Geometry: final body of the model. Coordinates: model frame, mm. Face numbers are marked on the shaded views. A direction names the side the tool comes from. Give positions to 0.01 mm unless a question says otherwise; leave off trailing zeros. Order: outer loops, then holes, each group sorted by start corner. A loop starts at its lowest first (then second) coordinate and runs counter-clockwise, first axis right, second up. Notation, with made-up numbers: (30, -13) -> (48, -13) arc R10 cw to (48, -7) -> close; hole circle Ø8 at (79, -24.75). An arc over 180 degrees is marked (long way). One line per item, written item: value. Start each with the question number.
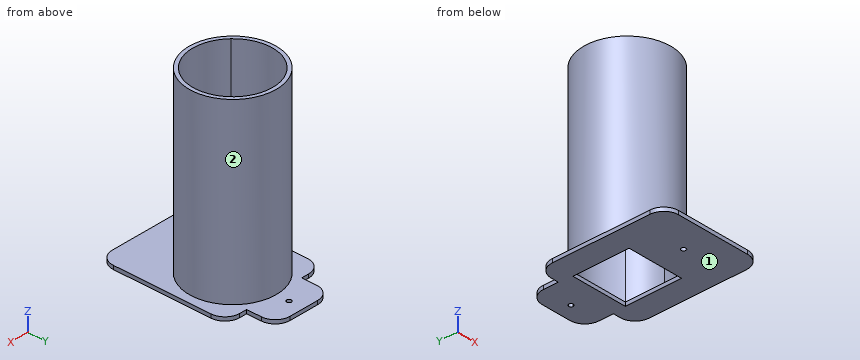
```python
from build123d import *

# Parameters (mm, degrees)
F0_W     = 24.13
F0_H     = 24.13
F0_W_2   = 44.45
F0_H_2   = 19.05
F0_R     = 1.016
F1_DEPTH = 1.5875
F2_R     = 6.35
F3_R     = 18.649987
F4_DEPTH = 76.2


with BuildPart() as f1:
    # F0 (on Top) → F1 (new body)
    with BuildSketch(Plane.XY):
        with BuildLine():
            Line((0, 17.78), (12.7, 17.78))
            Line((12.7, 17.78), (12.7, 30.48))
            Line((12.7, 30.48), (0, 30.48))
            Line((0, 30.48), (0, 25.146))
            ThreePointArc((0, 25.146), (0.71842, 24.84842), (1.016, 24.13))
            ThreePointArc((1.016, 24.13), (0.71842, 23.41158), (0, 23.114))
            Line((0, 23.114), (0, 17.78))
        make_face()
        with BuildLine():
            Line((-12.7, 30.48), (-12.7, 17.78))
            Line((-12.7, 17.78), (0, 17.78))
            Line((0, 17.78), (0, 23.114))
            ThreePointArc((0, 23.114), (-1.016, 24.13), (0, 25.146))
            Line((0, 25.146), (0, 30.48))
            Line((0, 30.48), (-12.7, 30.48))
        make_face()
        Polygon((-22.225, -17.78), (22.225, -17.78), (22.225, 17.78), (12.7, 17.78), (0, 17.78), (-12.7, 17.78), (-22.225, 17.78), align=None)
        Rectangle(F0_W, F0_H, mode=Mode.SUBTRACT)
        with Locations((0, -27.305)):
            Rectangle(F0_W_2, F0_H_2)
        with Locations((0, -24.13)):
            Circle(F0_R, mode=Mode.SUBTRACT)
    extrude(amount=F1_DEPTH)

    # F2
    f2_edges = [f1.edges().sort_by_distance(p)[0] for p in [
        (-12.7, 30.48, 0.79375),
        (-22.225, 17.78, 0.79375),
        (12.7, 30.48, 0.79375),
        (22.225, 17.78, 0.79375),
        (22.225, -36.83, 0.79375),
        (-22.225, -36.83, 0.79375),
    ]]
    fillet(f2_edges, radius=F2_R)

    # F3 (on face) → F4 (join)
    with BuildSketch(Plane.XY.offset(1.5875)):
        Circle(F3_R)
        with BuildLine():
            ThreePointArc((12.065, 12.065), (15.763682, 6.529531), (17.062487, 0))
            ThreePointArc((17.062487, 0), (15.763682, -6.529531), (12.065, -12.065))
            ThreePointArc((12.065, -12.065), (0, -17.062487), (-12.065, -12.065))
            ThreePointArc((-12.065, -12.065), (-17.062487, 0), (-12.065, 12.065))
            ThreePointArc((-12.065, 12.065), (0, 17.062487), (12.065, 12.065))
        make_face(mode=Mode.SUBTRACT)
    extrude(amount=F4_DEPTH)


solid = f1.part
```
1. Cut plane C-C, the plane z = 22. Return loops of the section in (x, y) (1 decimal), then the cut area to 3 significant figures.
2. Cut plane D-D, the plane y = 9.5. Return loops of the section in (x, z) (1 decimal), then the cut area to 3 significant figures.
3. Pin query (flat end, axial travel): P1, Ø2.5, axis at x = -14, y = 4, coming from the +Z side; P2, Ø0.8, axis at y = 21, z = 1, coming from the +X side; P3, Ø8, axis at y = -10, z = 47, coming from the -X side. Return the tip coordinate at first contact, or that it passes through.
4. Material intervals for L1, parallel to Y at x = 0, z = 0.4 (3 decimals); L2, parallel to Y at x = 0, z = 25; L3, parallel to Z at x = -15, y = -19, sorted ascending. Write a range as [from, to].
5. Cut plane B-B, the plane x = 5. Return loops of the section in (y, z) (1 decimal).
6. Access query for the marked faces 1 and 2. Directions: +Z, -Z, +X, -X, +Y, -Y. A direction counts if a zero-diameter tool reaches every point of the face in a straight line with its end or side. Return the directions, or none.
7. Cut plane A-A, the plane y = -24.13. Return loops of the section in (x, z) (1 decimal).
Answers follow:
1. outline: circle Ø37.3 at (0, 0); hole (-12.1, -12.1) arc R17.1 ccw to (12.1, -12.1) arc R17.1 ccw to (17.1, 0) arc R17.1 ccw to (12.1, 12.1) arc R17.1 ccw to (-12.1, 12.1) arc R17.1 ccw to start
1. area: 178 mm²
2. outline: (-22.2, 0) -> (-12.1, 0) -> (-12.1, 1.6) -> (-14.2, 1.6) -> (-14.2, 77.8) -> (-16, 77.8) -> (-16, 1.6) -> (-22.2, 1.6) -> close; (12.1, 0) -> (22.2, 0) -> (22.2, 1.6) -> (16, 1.6) -> (16, 77.8) -> (14.2, 77.8) -> (14.2, 1.6) -> (12.1, 1.6) -> close
2. area: 318 mm²
3. P1: stops at z = 1.59
3. P2: stops at x = 12.7
3. P3: stops at x = -17.66
4. L1: y = [-36.83, -25.146], [-23.114, -12.065], [12.065, 23.114], [25.146, 30.48]
4. L2: y = [-18.65, -17.06], [17.06, 18.65]
4. L3: z = [0, 1.59]
5. outline: (-36.8, 0) -> (-12.1, 0) -> (-12.1, 1.6) -> (-16.3, 1.6) -> (-16.3, 77.8) -> (-18, 77.8) -> (-18, 1.6) -> (-36.8, 1.6) -> close; (12.1, 0) -> (30.5, 0) -> (30.5, 1.6) -> (18, 1.6) -> (18, 77.8) -> (16.3, 77.8) -> (16.3, 1.6) -> (12.1, 1.6) -> close
6. face 1: -Z, +X, -X, +Y, -Y
6. face 2: +Z
7. outline: (-22.2, 0) -> (-1, 0) -> (-1, 1.6) -> (-22.2, 1.6) -> close; (1, 0) -> (22.2, 0) -> (22.2, 1.6) -> (1, 1.6) -> close
